Geometry: see drawing. Coordinates: mm, zero at the bounding-box minimum. A direction names the side the tool comes from. Coordinates: 2 decimals unless noted, no trailing zeros. Order: outer loops, then holes, each group sorted by start corner. A loop starts at its lowest first (then second) coordinate and runs counter-clockwise, first axis right, second up.
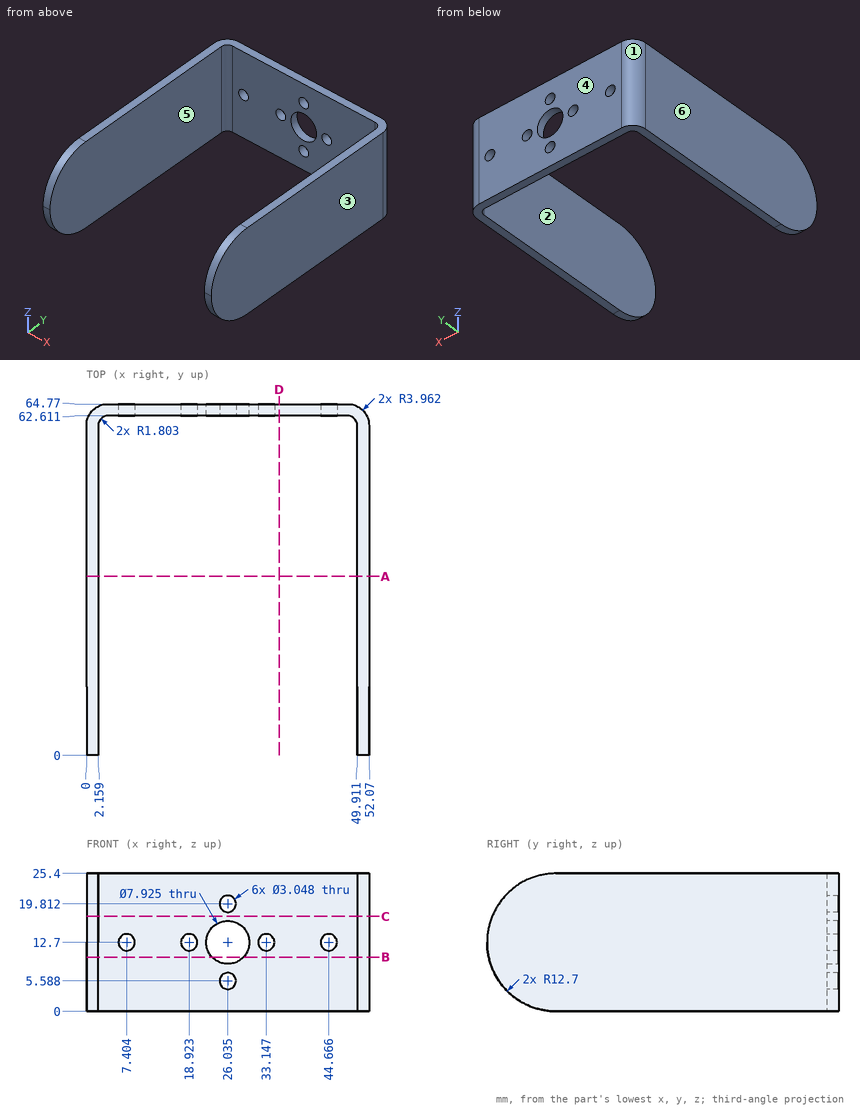
Item 1: Draft query along X for the marked faces 3, 4, 5 and 6. Return one class per face: pulls with the +X half, pulls with the -X half, needs draft (parallel to the pull), parting line crosses it, or undercut.
Response values:
face 3: pulls with the +X half
face 4: needs draft
face 5: undercut
face 6: pulls with the -X half
Item 2: Ray query, probe 1 along X at (y, z) = (49, 4.25); probe 2 along Y at (x, z) = (8, 8.5); probe 3 along Y at (x, z) = (49, 23) (1 decimal). Return the intervals inside material, ascending.
Response values:
probe 1: x = 0 to 2.16, 49.91 to 52.07
probe 2: y = 62.61 to 64.77
probe 3: y = 62.4 to 64.7
Item 3: Pin query (flat end, axial travel): pin 1 Ø3.5 at (x, z) = (26.035, 5.588) entering from -Y; pin 2 Ø2.5 at (x, z) = (18.923, 12.7) entering from +Y. Return the tip coordinate at first contact, or that it passes through.
Response values:
pin 1: stops at y = 62.61
pin 2: passes through
Item 4: Access query for the marked faces 1 and 2. Directions: +Z, -Z, +X, -X, +Y, -Y. A direction counts if a zero-diameter tool reaches every point of the face in a straight line with its end or side. Return the directions, or none.
Response values:
face 1: +Z, -Z, -X, +Y
face 2: +Z, -Z, -Y
Item 5: Cut plane B-B on z = 10. Return loops of the section in (x, y) (1 decimal).
Response values:
outline: (0, 0.3) - (2.2, 0.3) - (2.2, 60.8) arc R1.8 cw to (4, 62.6) - (23.1, 62.6) - (23.1, 64.8) - (4, 64.8) arc R4 ccw to (0, 60.8) - close; (28.9, 62.6) - (48.1, 62.6) arc R1.8 cw to (49.9, 60.8) - (49.9, 0.3) - (52.1, 0.3) - (52.1, 60.8) arc R4 ccw to (48.1, 64.8) - (28.9, 64.8) - close
Item 6: Cut plane C-C on z = 17.5. Return loops of the section in (x, y) (1 decimal).
Response values:
outline: (0, 0.9) - (2.2, 0.9) - (2.2, 60.8) arc R1.8 cw to (4, 62.6) - (48.1, 62.6) arc R1.8 cw to (49.9, 60.8) - (49.9, 0.9) - (52.1, 0.9) - (52.1, 60.8) arc R4 ccw to (48.1, 64.8) - (4, 64.8) arc R4 ccw to (0, 60.8) - close
Item 7: Cut plane D-D on x = 35.5. Return loops of the section in (y, z).
Response values:
outline: (62.61, 0) - (64.77, 0) - (64.77, 25.4) - (62.61, 25.4) - close
Item 8: Cut plane A-A on y = 33. Return loops of the section in (x, z), then the cut area to 3 significant figures.
Response values:
outline: (0, 0) - (2.16, 0) - (2.16, 25.4) - (0, 25.4) - close; (49.91, 0) - (52.07, 0) - (52.07, 25.4) - (49.91, 25.4) - close
area: 110 mm2
